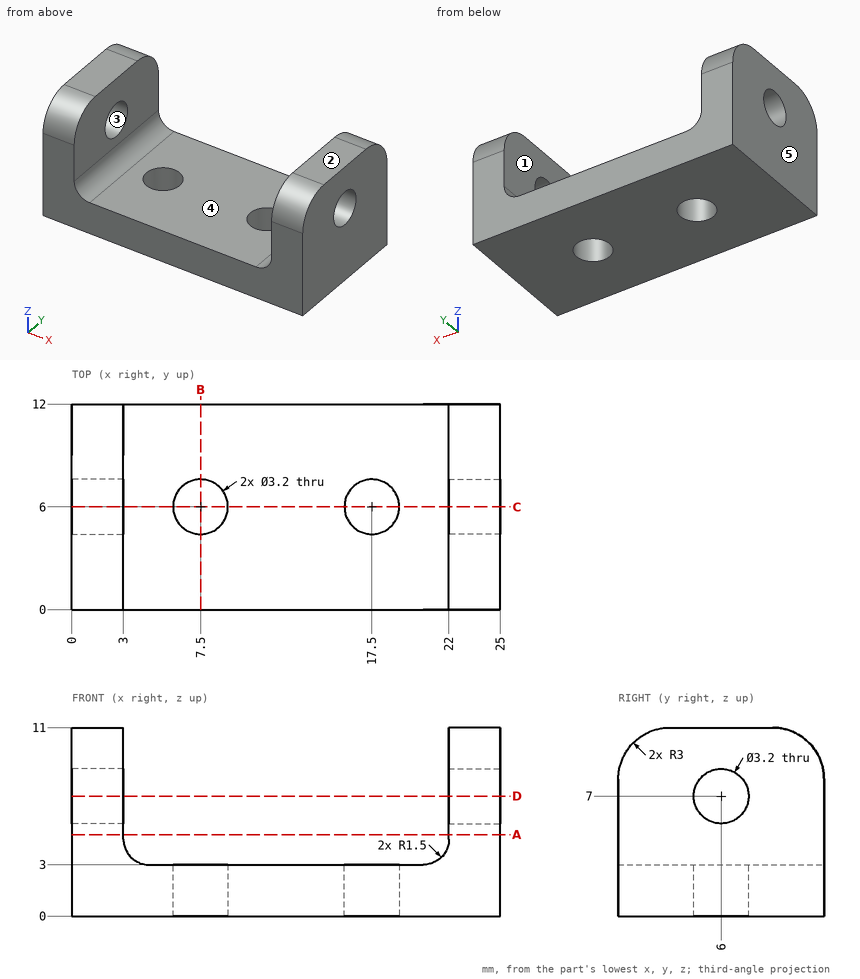
Input: dimensioned drawing with shaded views. Units: mm. Origin: part minimum x, y, z. A direction names the side the tool comes from. Round coordinates to 2 decimals unless told otherwise and drop trailing zeros. Loops run counter-clockwise (first coordinate to the right, second up) from the corner with the lowest first, then second, coordinate; pieces in that order, holes last.
1) Section query C-C on y = 6. Return the cut outline in (x, z), plus the area to 3 significant figures.
Ans:
outline: (0, 0) - (5.9, 0) - (5.9, 3) - (4.5, 3) arc R1.5 cw to (3, 4.5) - (3, 5.4) - (0, 5.4) - close; (0, 8.6) - (3, 8.6) - (3, 11) - (0, 11) - close; (9.1, 0) - (15.9, 0) - (15.9, 3) - (9.1, 3) - close; (19.1, 0) - (25, 0) - (25, 5.4) - (22, 5.4) - (22, 4.5) arc R1.5 cw to (20.5, 3) - (19.1, 3) - close; (22, 8.6) - (25, 8.6) - (25, 11) - (22, 11) - close
area: 85.6 mm2
2) Pin query (flat end, axial travel): pin 1 (6 mm diameter, centred on x = 16.5, z = 9, fed in from +Y); pin 2 (4 mm diameter, centred on y = 6, z = 7, fed in from -X); pin 3 (5 mm diameter, centred on x = 17.5, y = 6, fed in from +Z). Return the tip coordinate at first contact, or that it passes through.
Ans:
pin 1: passes through
pin 2: stops at x = 0
pin 3: stops at z = 3
3) Section query A-A on z = 4.75. Return the cut outline in (x, y).
Ans:
outline: (0, 0) - (3, 0) - (3, 12) - (0, 12) - close; (22, 0) - (25, 0) - (25, 12) - (22, 12) - close
4) Set-up query: the marked faces 1 and 2. Return all of +Z, -Z, +X, -X, +Y, -Y with unobstructed straight access to the full face (end or side cutting, diameter ignored); none if empty.
Ans:
face 1: +Z, +Y, -Y
face 2: +Z, +X, -X, +Y, -Y
5) Section query D-D on z = 7. Return the cut outline in (x, y).
Ans:
outline: (0, 0) - (3, 0) - (3, 4.4) - (0, 4.4) - close; (0, 7.6) - (3, 7.6) - (3, 12) - (0, 12) - close; (22, 0) - (25, 0) - (25, 4.4) - (22, 4.4) - close; (22, 7.6) - (25, 7.6) - (25, 12) - (22, 12) - close
6) Section query B-B on x = 7.5. Return the cut outline in (y, z), plus the area to 3 significant figures.
Ans:
outline: (0, 0) - (4.4, 0) - (4.4, 3) - (0, 3) - close; (7.6, 0) - (12, 0) - (12, 3) - (7.6, 3) - close
area: 26.4 mm2
7) Pull-direction query (Z, two-part tool) for the marked faces 3, 4 and 5; classes: released by +Z, released by -Z, zero draft, split by the parting line, or undercut.
Ans:
face 3: undercut
face 4: released by +Z
face 5: zero draft
8) Material intervals for line 1 (X direction, y = 2.75, z = 5); line 2 (Y direction, x = 7.5, z = 1.1); line 3 (X direction, y = 7, z = 1.5), sorted ascending.
Ans:
line 1: x = 0 to 3, 22 to 25
line 2: y = 0 to 4.4, 7.6 to 12
line 3: x = 0 to 6.25, 8.75 to 16.25, 18.75 to 25
